```python
from build123d import *

# Parameters (mm, degrees)
BOSS_EXTRUDE1_DEPTH = 304.8
SKETCH4_W           = 12.7
SKETCH4_H           = 6.223
CUT_EXTRUDE1_DEPTH  = 306.114409233
LPATTERN1_COUNT     = 24
LPATTERN1_PITCH     = 25.4
BOSS_EXTRUDE2_DEPTH = 609.6
SKETCH6_W           = 12.7
SKETCH6_H           = 6.223
CUT_EXTRUDE2_DEPTH  = 306.114409233
LPATTERN2_COUNT     = 24
LPATTERN2_PITCH     = 25.4
SKETCH7_R           = 1.5875
BOSS_EXTRUDE3_DEPTH = 609.6
CHAMFER1_SIZE       = 0.3175
CUT_EXTRUDE3_START  = -88.9
SKETCH8_W           = 11.762471384
SKETCH8_H           = 30.066276354
CUT_EXTRUDE3_DEPTH  = 521.857265411
FILLET1_R           = 3.175
SKETCH9_R           = 2.032
SKETCH9_R_2         = 2.031999998
CUT_EXTRUDE4_DEPTH  = 306.162001268


with BuildPart() as part:
    # Sketch3 → Boss-Extrude1 (new, symmetric)
    with BuildSketch(Plane(origin=(0, 0, 0), x_dir=(0, 0, -1), z_dir=(1, 0, 0))):
        with BuildLine():
            Line((1.5875, 0), (1.5875, -2.676056053))
            Line((1.5875, -2.676056053), (1.5875, -13.49375))
            Line((1.5875, -13.49375), (3.1115, -13.49375))
            Line((3.1115, -13.49375), (3.1115, 0))
            ThreePointArc((3.1115, 0), (-2.624212484, 1.671807731), (1.314976721, -2.819976679))
            Line((1.314976721, -2.819976679), (0.670906491, -1.438763612))
            ThreePointArc((0.670906491, -1.438763612), (-1.33888392, 0.852963128), (1.5875, 0))
        make_face()
    extrude(amount=BOSS_EXTRUDE1_DEPTH, both=True)

    # Sketch4 → Cut-Extrude1 (cut, symmetric)
    with BuildSketch(Plane.XY):
        with Locations((298.45, 0)):
            Rectangle(SKETCH4_W, SKETCH4_H)
    cut_extrude1 = extrude(amount=CUT_EXTRUDE1_DEPTH, both=True, mode=Mode.SUBTRACT)

    # LPattern1: Cut-Extrude1 ×24
    with Locations(*[(-i * LPATTERN1_PITCH, 0, 0) for i in range(1, LPATTERN1_COUNT)]):
        add(cut_extrude1, mode=Mode.SUBTRACT)


with BuildPart() as body_2:
    # Sketch5 → Boss-Extrude2 (new body)
    with BuildSketch(Plane(origin=(304.8, 0, 0), x_dir=(0, 0, -1), z_dir=(1, 0, 0))):
        with BuildLine():
            Line((1.5875, 13.49375), (1.5875, 2.676056053))
            Line((1.5875, 2.676056053), (1.5875, 0))
            ThreePointArc((1.5875, 0), (-1.33888392, -0.852963128), (0.670906491, 1.438763612))
            Line((0.670906491, 1.438763612), (1.314976721, 2.819976679))
            ThreePointArc((1.314976721, 2.819976679), (-2.624212484, -1.671807731), (3.1115, 0))
            Line((3.1115, 0), (3.1115, 13.49375))
            Line((3.1115, 13.49375), (1.5875, 13.49375))
        make_face()
    extrude(amount=-BOSS_EXTRUDE2_DEPTH)

    # Sketch6 → Cut-Extrude2 (cut, symmetric)
    with BuildSketch(Plane.XY):
        with Locations((285.75, 0)):
            Rectangle(SKETCH6_W, SKETCH6_H)
    cut_extrude2 = extrude(amount=CUT_EXTRUDE2_DEPTH, both=True, mode=Mode.SUBTRACT)

    # LPattern2: Cut-Extrude2 ×24
    with Locations(*[(-i * LPATTERN2_PITCH, 0, 0) for i in range(1, LPATTERN2_COUNT)]):
        add(cut_extrude2, mode=Mode.SUBTRACT)


with BuildPart() as body_3:
    # Sketch7 → Boss-Extrude3 (new body)
    with BuildSketch(Plane(origin=(304.8, 0, 0), x_dir=(0, 0, -1), z_dir=(1, 0, 0))):
        Circle(SKETCH7_R)
    extrude(amount=-BOSS_EXTRUDE3_DEPTH)

    # Chamfer1
    chamfer1_edges = [body_3.edges().sort_by_distance(p)[0] for p in [
        (304.8, 0, 1.5875),
        (-304.8, 0, 1.5875),
    ]]
    chamfer(chamfer1_edges, length=CHAMFER1_SIZE)


with BuildPart() as cut_extrude3_tool:
    # Sketch8 → Cut-Extrude3 (new, through all)
    with BuildSketch(Plane.ZY.offset(304.8).offset(CUT_EXTRUDE3_START)):
        Rectangle(SKETCH8_W, SKETCH8_H)
    extrude(amount=-CUT_EXTRUDE3_DEPTH)


with BuildPart() as part_1:
    add(part.part)

    # Cut-Extrude3: cut by cut_extrude3_tool
    add(cut_extrude3_tool.part, mode=Mode.SUBTRACT)


with BuildPart() as body_2_1:
    add(body_2.part)

    # Cut-Extrude3: cut by cut_extrude3_tool
    add(cut_extrude3_tool.part, mode=Mode.SUBTRACT)

    # Fillet1
    fillet1_edges = [body_2_1.edges().sort_by_distance(p)[0] for p in [
        (-304.8, 13.49375, -2.3495),
        (-215.9, 13.49375, -2.3495),
    ]]
    fillet(fillet1_edges, radius=FILLET1_R)

    # Sketch9 → Cut-Extrude4 (cut, through all)
    with BuildSketch(Plane(origin=(0, 0, -3.1115), x_dir=(-1, 0, 0), z_dir=(0, 0, -1))):
        with Locations(Location((228.600000002, 7.874000002, 0), (0, 0, 90))):
            Circle(SKETCH9_R)
        with Locations(Location((292.100000002, 7.874000002, 0), (0, 0, 90))):
            Circle(SKETCH9_R_2)
    extrude(amount=-CUT_EXTRUDE4_DEPTH, mode=Mode.SUBTRACT)


with BuildPart() as body_3_1:
    add(body_3.part)

    # Cut-Extrude3: cut by cut_extrude3_tool
    add(cut_extrude3_tool.part, mode=Mode.SUBTRACT)


solid = body_2_1.part
```
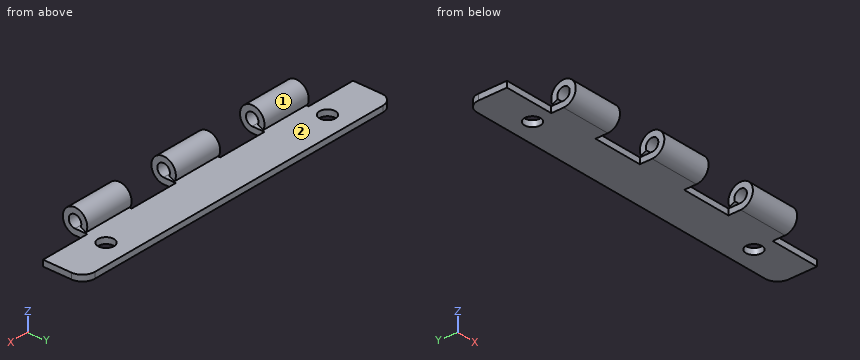
Check sheet for the modelled part. Datum: model origin and axes. Units: mm. Face numbers are marked on the shaded views. A direction names the side the tool comes from. Round coordinates to 2 decimals unless told otherwise and drop trailing zeros. Order: outer loops, then holes, each group sorted by start corner. A loop starts at its lowest first (then second) coordinate and runs counter-clockwise, first axis right, second up. Notation, with made-up numbers: (-3.5, 20) - (55.5, 20) arc R18 cw to (55.5, 43) - close; hole circle Ø10 at (25.25, 64.25). An arc over 180 degrees is marked (long way). Write item = value, one per line.
Q1. Tool access check on the marked faces 1 and 2. Record the directions out of +Z, -Z, +X, -X, +Y, -Y that give a thin tool (end or side, any length) a straight path to the whole face; none if there is none.
Computed:
face_1 = +X, -X
face_2 = +X, -X, +Y
Q2. Go/stop test with flat-tipped pins: pin 1 (0.5 mm diameter, centred on x = -225, z = -2, fed in from -Y); pin 2 (3 mm diameter, centred on y = -0.5, z = 0, fed in from -X); pin 3 (5 mm diameter, centred on x = -270.5, y = -1.5, fed in from +Z); pin 4 (1 mm diameter, centred on x = -248.5, y = 3, fed in from +Z). Record where each tip stops, or that it passes through.
Computed:
pin_1 = 3.11
pin_2 = -292.1
pin_3 = through
pin_4 = -1.59
Q3. Section check B-B (y = 4). Record the boundary of the cut face in (x, z), and give its area (3 significant figures).
Computed:
outline = (-304.8, -3.11) - (-215.9, -3.11) - (-215.9, -1.59) - (-304.8, -1.59) - close
area = 135 mm^2
Q4. Section check A-A (x = -235). Record the boundary of the cut face in (y, z) (1 decimal).
Computed:
outline = (0, -3.1) - (13.5, -3.1) - (13.5, -1.6) - (0, -1.6) arc R1.6 cw (long way) to (1.4, -0.7) - (2.8, -1.3) arc R3.1 ccw (long way) to start
Q5. Thickness scan on line 1 along X through (y, z) = (2.25, 2); line 2 along Y through (x, z) = (-281.75, 0). Record the ranges inside material, lowest first.
Computed:
line_1 = -292.1 to -279.4, -266.7 to -254, -241.3 to -228.6
line_2 = -3.11 to -1.59, 1.59 to 3.11
Q6. Section check C-C (x = -249). Record the boundary of the cut face in (y, z).
Computed:
outline = (3.11, -3.11) - (13.49, -3.11) - (13.49, -1.59) - (3.11, -1.59) - close
